from build123d import *

# Parameters (mm, degrees)
CROQUIS1_R              = 1.6
CROQUIS1_R_2            = 1.65
CROQUIS1_W              = 95
CROQUIS1_H              = 68.859019413
CROQUIS1_R_3            = 1.5
CROQUIS1_W_2            = 59.75
SALIENTE_EXTRUIR2_DEPTH = 1.5
CROQUIS4_R              = 3
CROQUIS4_R_2            = 4
SALIENTE_EXTRUIR3_DEPTH = 7.6
CORTAR_EXTRUIR2_START   = -17.6
CROQUIS5_R              = 1.6
CROQUIS5_R_2            = 1.5
CORTAR_EXTRUIR2_DEPTH   = 17.6


with BuildPart() as part:
    # Croquis1 → Saliente-Extruir2 (new body)
    with BuildSketch(Plane(origin=(0, 0, 0), x_dir=(1, 0, 0), z_dir=(0, 1, 0))):
        Polygon((-81.153068025, 81.276875237), (-81.153068025, -81.723124763), (46.345958321, -81.723124763), (46.345958321, -56.5), (81.846931975, -56.5), (81.846931975, 81.276875237), align=None)
        with Locations(Location((-69.2, -69.3, 0), (0, 0, 270))):
            Circle(CROQUIS1_R, mode=Mode.SUBTRACT)
        with Locations(Location((-35, -78.25, 0), (0, 0, 270))):
            Circle(CROQUIS1_R_2, mode=Mode.SUBTRACT)
        with Locations(Location((0, -78.25, 0), (0, 0, 270))):
            Circle(CROQUIS1_R_2, mode=Mode.SUBTRACT)
        with Locations(Location((-78.25, -35, 0), (0, 0, 270))):
            Circle(CROQUIS1_R_2, mode=Mode.SUBTRACT)
        with Locations(Location((-69.2, -13.2, 0), (0, 0, 270))):
            Circle(CROQUIS1_R, mode=Mode.SUBTRACT)
        with Locations((-16.5, -39.570490294)):
            Rectangle(CROQUIS1_W, CROQUIS1_H, mode=Mode.SUBTRACT)
        with Locations(Location((35, -78.25, 0), (0, 0, 270))):
            Circle(CROQUIS1_R_2, mode=Mode.SUBTRACT)
        with Locations(Location((36.7, -69.3, 0), (0, 0, 270))):
            Circle(CROQUIS1_R, mode=Mode.SUBTRACT)
        with Locations(Location((52.645958321, -49.9, 0), (0, 0, 270))):
            Circle(CROQUIS1_R_3, mode=Mode.SUBTRACT)
        with Locations(Location((36.7, -13.6, 0), (0, 0, 270))):
            Circle(CROQUIS1_R, mode=Mode.SUBTRACT)
        with Locations(Location((78.25, -35, 0), (0, 0, 270))):
            Circle(CROQUIS1_R_2, mode=Mode.SUBTRACT)
        with Locations(Location((68.845958321, -20, 0), (0, 0, 270))):
            Circle(CROQUIS1_R_3, mode=Mode.SUBTRACT)
        with Locations(Location((-78.25, 0, 0), (0, 0, 270))):
            Circle(CROQUIS1_R_2, mode=Mode.SUBTRACT)
        with Locations(Location((-70, 1.359281772, 0), (0, 0, 270))):
            Circle(CROQUIS1_R_3, mode=Mode.SUBTRACT)
        with Locations(Location((-78.25, 35, 0), (0, 0, 270))):
            Circle(CROQUIS1_R_2, mode=Mode.SUBTRACT)
        with Locations(Location((-2, 1.359281772, 0), (0, 0, 270))):
            Circle(CROQUIS1_R_3, mode=Mode.SUBTRACT)
        Polygon((-74, 62.876032496), (-65, 62.876032496), (-65, 73.859019413), (4.25, 73.859019413), (4.25, 6.359281772), (-65, 6.359281772), (-74, 6.359281772), align=None, mode=Mode.SUBTRACT)
        with Locations(Location((-70, 67.859019413, 0), (0, 0, 270))):
            Circle(CROQUIS1_R_3, mode=Mode.SUBTRACT)
        with Locations(Location((-35, 78.25, 0), (0, 0, 270))):
            Circle(CROQUIS1_R_2, mode=Mode.SUBTRACT)
        with Locations(Location((0, 78.25, 0), (0, 0, 270))):
            Circle(CROQUIS1_R_2, mode=Mode.SUBTRACT)
        with Locations(Location((9.25, 0, 0), (0, 0, 270))):
            Circle(CROQUIS1_R_3, mode=Mode.SUBTRACT)
        with Locations(Location((78.25, 0, 0), (0, 0, 270))):
            Circle(CROQUIS1_R_2, mode=Mode.SUBTRACT)
        with Locations((44.125, 39.429509706)):
            Rectangle(CROQUIS1_W_2, CROQUIS1_H, mode=Mode.SUBTRACT)
        with Locations(Location((78.25, 35, 0), (0, 0, 270))):
            Circle(CROQUIS1_R_2, mode=Mode.SUBTRACT)
        with Locations(Location((9.25, 63.5, 0), (0, 0, 270))):
            Circle(CROQUIS1_R_3, mode=Mode.SUBTRACT)
        with Locations(Location((35, 78.25, 0), (0, 0, 270))):
            Circle(CROQUIS1_R_2, mode=Mode.SUBTRACT)
        with Locations(Location((78.25, 76.999306834, 0), (0, 0, 270))):
            Circle(CROQUIS1_R_3, mode=Mode.SUBTRACT)
    extrude(amount=SALIENTE_EXTRUIR2_DEPTH)

    # Croquis4 → Saliente-Extruir3 (add)
    with BuildSketch(Plane.XZ):
        with Locations(Location((-69.2, 69.3, 0), (0, 0, 90))):
            Circle(CROQUIS4_R)
        with Locations(Location((-69.2, 13.2, 0), (0, 0, 90))):
            Circle(CROQUIS4_R)
        with Locations(Location((36.7, 13.6, 0), (0, 0, 90))):
            Circle(CROQUIS4_R)
        with Locations(Location((52.645958321, 49.9, 0), (0, 0, 90))):
            Circle(CROQUIS4_R)
        with Locations(Location((68.845958321, 20, 0), (0, 0, 90))):
            Circle(CROQUIS4_R)
        with Locations(Location((9.25, 0, 0), (0, 0, 90))):
            Circle(CROQUIS4_R)
        with Locations(Location((-2, -1.359281772, 0), (0, 0, 90))):
            Circle(CROQUIS4_R)
        with Locations(Location((-70, -1.359281772, 0), (0, 0, 90))):
            Circle(CROQUIS4_R)
        with Locations(Location((-70, -67.859019413, 0), (0, 0, 90))):
            Circle(CROQUIS4_R_2)
        with Locations(Location((9.25, -63.5, 0), (0, 0, 90))):
            Circle(CROQUIS4_R)
        with Locations(Location((78.25, -76.999306834, 0), (0, 0, 90))):
            Circle(CROQUIS4_R)
        with Locations(Location((36.7, 69.3, 0), (0, 0, 90))):
            Circle(CROQUIS4_R)
    extrude(amount=SALIENTE_EXTRUIR3_DEPTH)

    # Croquis5 → Cortar-Extruir2 (cut)
    with BuildSketch(Plane(origin=(0, 1.5, 0), x_dir=(1, 0, 0), z_dir=(0, 1, 0)).offset(CORTAR_EXTRUIR2_START)):
        with Locations(Location((-69.2, -13.2, 0), (0, 0, 90))):
            Circle(CROQUIS5_R)
        with Locations(Location((-70, 1.359281772, 0), (0, 0, 90))):
            Circle(CROQUIS5_R_2)
        with Locations(Location((-2, 1.359281772, 0), (0, 0, 90))):
            Circle(CROQUIS5_R_2)
        with Locations(Location((9.25, 0, 0), (0, 0, 90))):
            Circle(CROQUIS5_R_2)
        with Locations(Location((36.7, -13.6, 0), (0, 0, 90))):
            Circle(CROQUIS5_R)
        with Locations(Location((36.7, -69.3, 0), (0, 0, 90))):
            Circle(CROQUIS5_R)
        with Locations(Location((52.645958321, -49.9, 0), (0, 0, 90))):
            Circle(CROQUIS5_R_2)
        with Locations(Location((68.845958321, -20, 0), (0, 0, 90))):
            Circle(CROQUIS5_R_2)
        with Locations(Location((9.25, 63.5, 0), (0, 0, 270))):
            Circle(CROQUIS5_R)
        with Locations(Location((-70, 67.859019413, 0), (0, 0, 270))):
            Circle(CROQUIS5_R)
        with Locations(Location((-69.2, -69.3, 0), (0, 0, 90))):
            Circle(CROQUIS5_R)
        with Locations(Location((78.25, 76.999306834, 0), (0, 0, 90))):
            Circle(CROQUIS5_R_2)
    extrude(amount=CORTAR_EXTRUIR2_DEPTH, mode=Mode.SUBTRACT)


solid = part.part
Can you work these out from the model? Positions are in its coordinate system, mm. A direction names the side the tool comes from. Coordinates: 2 decimals unless noted, no trailing zeros. Write each loop counter-clockwise with the first axis right and the second up, starting at its lowest first coordinate (ties: lowest second). Pieces come first, ordered by that corner, then holes. Notation, with made-up numbers: (51, -24.75) - (66, -24.75) arc R11 cw to (66, -18.75) - close; hole circle Ø6 at (43.5, -6.75). An arc over 180 degrees is marked (long way). Return JSON: item names as keys, results as strings. Group by question number.
Item 1: Please list where these lines run through material, in increasing order: probe 1 along Z at (x, y) = (-21.5, 0.5); probe 2 along Z at (x, y) = (78.25, 0.95); probe 3 along X at (y, z) = (0.4, -35).
Item 2: We'd pull the mould along Z, two halves only. Please class faces 3 (the face through (-66.451, -3.747, -66.013)), 4 (the face through (55.575, -3.747, 49.25)), 5 (the face through (34.67, -3.75, 11.39)), 6 (the face through (-69, -7.6, -3)): pulls with the +Z half, pulls with the -Z half, needs draft (parallel to the pull), parting line crosses it, or undercut.
Item 3: If we section it at A-A (x = -62): Write out the boundary of the cut face in (y, z).
Item 4: I'm going to push flat-ended pins straight in: pin 1 Ø2 at (x, y) = (12, -6) entering from -Z; pin 2 Ø2.5 at (x, z) = (-69.2, 13.2) entering from +Y; pin 3 Ø3.5 at (x, z) = (9.25, -63.5) entering from +Y; pin 4 Ø1.6 at (y, z) = (0.5, 67) entering from +X. Where does each tip first touch, or does it pass through?
Item 5: If we section it at C-C (z = -18.5): Write out the boundary of the cut face in (x, y), then the cut area to 3 significant figures.
Item 6: Which directions (+Z, -Z, +X, -X, +Y, -Y) give clear straight access to the entire face, cutting with the end or side of a thin tool? Please do faces 1 (the face through (-66.538, -3.747, 14.584)), 2 (the face through (51, -7.6, 51)).
Item 7: If we section it at D-D (x = 44): Write out the boundary of the cut face in (y, z).
Item 8: If we section it at B-B (y = -4.25): Count the separate pieces of the cut face and the enclosed holes in it, then the cut area to 3 significant figures.
Return value:
{
 "1": {"probe 1": "z = -81.28 to -73.86, -6.36 to 5.14, 74 to 81.72", "probe 2": "z = -81.28 to -78.5, -75.5 to -36.65, -33.35 to -1.65, 1.65 to 33.35, 36.65 to 56.5", "probe 3": "x = -81.15 to -79.9, -76.6 to -74, 4.25 to 14.25, 74 to 76.6, 79.9 to 81.85"},
 "2": {"face 3": "undercut", "face 4": "parting line crosses it", "face 5": "undercut", "face 6": "needs draft"},
 "3": {"outline": "(0, -81.28) - (1.5, -81.28) - (1.5, -73.86) - (0, -73.86) - close; (0, -6.36) - (1.5, -6.36) - (1.5, 5.14) - (0, 5.14) - close; (0, 74) - (1.5, 74) - (1.5, 81.72) - (0, 81.72) - close"},
 "4": {"pin 1": "stops at z = -65.94", "pin 2": "passes through", "pin 3": "stops at y = 1.5", "pin 4": "stops at x = 46.35"},
 "5": {"outline": "(-81.15, 0) - (-74, 0) - (-74, 1.5) - (-81.15, 1.5) - close; (4.25, 0) - (14.25, 0) - (14.25, 1.5) - (4.25, 1.5) - close; (74, 0) - (81.85, 0) - (81.85, 1.5) - (74, 1.5) - close", "area": "37.5 mm^2"},
 "6": {"face 1": "-Y", "face 2": "+Z, -Z, +X, -X, -Y"},
 "7": {"outline": "(0, -81.28) - (1.5, -81.28) - (1.5, -73.86) - (0, -73.86) - close; (0, -5) - (1.5, -5) - (1.5, 81.72) - (0, 81.72) - close"},
 "8": {"separate pieces": "12", "enclosed holes": "12", "area": "271 mm^2"}
}
